from build123d import *

# Parameters (mm, degrees)
BOSS_EXTRUDE1_DEPTH        = 2
FILLET1_R                  = 2
F_2_9_2_9_DIAMETER_HOLE1_D = 2.9


with BuildPart() as part:
    # Sketch1 → Boss-Extrude1 (new body)
    with BuildSketch(Plane(origin=(0, 0, 0), x_dir=(1, 0, 0), z_dir=(0, 1, 0))):
        with BuildLine():
            Line((-32, 22.29349681), (-32, -22.29349681))
            ThreePointArc((-32, -22.29349681), (-7.038963606, -38.359522825), (22, -32.202484376))
            Line((22, -32.202484376), (22, 32.202484376))
            ThreePointArc((22, 32.202484376), (-7.038963606, 38.359522825), (-32, 22.29349681))
        make_face()
    extrude(amount=BOSS_EXTRUDE1_DEPTH)

    # Fillet1
    fillet1_edges = [part.edges().sort_by_distance(p)[0] for p in [
        (22, 1, -32.202484376),
        (22, 1, 32.202484376),
        (-32, 1, 22.29349681),
        (-32, 1, -22.29349681),
    ]]
    fillet(fillet1_edges, radius=FILLET1_R)

    # Ø2.9 (2.9) Diameter Hole1 (through all)
    with Locations(Plane(origin=(0, 2, 0), x_dir=(1, 0, 0), z_dir=(0, 1, 0))):
        with Locations((-28.5, 21.15), (-28.5, -21.15), (18.5, -30.3), (18.5, 30.3), (-5, 35.15), (-5, -35.15)):
            Hole(F_2_9_2_9_DIAMETER_HOLE1_D / 2)


solid = part.part
Read the model definition and answer for the solid it produces. Units are mm, in the model's axes. Round coordinates to 2 decimals unless told otherwise and drop trailing zeros. Write each loop counter-clockwise with the first axis right and the second up, starting at its lowest first coordinate (ties: lowest second). Pieces come first, ordered by that corner, then holes.
Q1. Find section D-D on x = -28.5. Determine the outline of the cut face in (y, z).
Values:
outline: (0, -26.62) - (2, -26.62) - (2, -22.6) - (0, -22.6) - close; (0, -19.7) - (2, -19.7) - (2, 19.7) - (0, 19.7) - close; (0, 22.6) - (2, 22.6) - (2, 26.62) - (0, 26.62) - close
Q2. The mould has two halves that part along X. Classify faces 1 (the face through (-4.686, 0.986, 36.566)), 2 (the face through (-5, 0, -1)), 3 (the face through (-32, 1, 0)), 4 (the face through (22, 1, 0)): released by +X, released by -X, zero draft, split by the parting line, or undercut.
Values:
face 1: undercut
face 2: zero draft
face 3: released by -X
face 4: released by +X
Q3. Find section C-C on x = -5. Determine the outline of the cut face in (y, z).
Values:
outline: (0, -38.68) - (2, -38.68) - (2, -36.6) - (0, -36.6) - close; (0, -33.7) - (2, -33.7) - (2, 33.7) - (0, 33.7) - close; (0, 36.6) - (2, 36.6) - (2, 38.68) - (0, 38.68) - close
Q4. Find section B-B on z = 30.3. Determine the outline of the cut face in (x, y).
Values:
outline: (-24.55, 0) - (17.05, 0) - (17.05, 2) - (-24.55, 2) - close; (19.95, 0) - (22, 0) - (22, 2) - (19.95, 2) - close
Q5. Straight lines are drawn through the part: line 1 (Z direction, x = -5, y = 1); line 2 (Z direction, x = 18.5, y = 0.9); line 3 (X direction, y = 0.4, z = -31). For each, find the intervals that lie inside material, in ascending order.
Values:
line 1: z = -38.68 to -36.6, -33.7 to 33.7, 36.6 to 38.68
line 2: z = -34.33 to -31.75, -28.85 to 28.85, 31.75 to 34.33
line 3: x = -23.66 to 17.23, 19.77 to 22
Q6. Find section A-A on y = 1.15. Determine the outline of the cut face in (x, z), and give its area (3 significant figures).
Values:
outline: (-32, -21.66) arc R2 ccw to (-31.62, -22.83) arc R39 ccw to (21.08, -32.81) arc R2 ccw to (22, -31.13) - (22, 31.13) arc R2 ccw to (21.08, 32.81) arc R39 ccw to (-31.62, 22.83) arc R2 ccw to (-32, 21.66) - close; hole circle Ø2.9 at (-28.5, -21.15); hole circle Ø2.9 at (-28.5, 21.15); hole circle Ø2.9 at (-5, -35.15); hole circle Ø2.9 at (-5, 35.15); hole circle Ø2.9 at (18.5, -30.3); hole circle Ø2.9 at (18.5, 30.3)
area: 3,760 mm2
